```python
from build123d import *

# Parameters (mm, degrees)
F0_W     = 1300
F0_H     = 600
F1_DEPTH = 800
F2_W     = 1220
F2_H     = 80
F3_DEPTH = 800.001
F4_W     = 1220
F4_H     = 200
F5_DEPTH = 800.001
F6_W     = 590
F6_H     = 200
F7_DEPTH = 780


with BuildPart() as f1:
    # F0 (on Front) → F1 (new body)
    with BuildSketch(Plane.XZ):
        Rectangle(F0_W, F0_H)
    extrude(amount=F1_DEPTH)

    # F2 (on face) → F3 (cut, through all)
    with BuildSketch(Plane.XZ.offset(800)):
        with Locations((0, -260)):
            Rectangle(F2_W, F2_H)
    extrude(amount=-F3_DEPTH, mode=Mode.SUBTRACT)

    # F4 (on face) → F5 (cut, through all)
    with BuildSketch(Plane.XZ.offset(800)):
        with Locations((0, 160)):
            Rectangle(F4_W, F4_H)
    extrude(amount=-F5_DEPTH, mode=Mode.SUBTRACT)

    # F6 (on face) → F7 (cut)
    with BuildSketch(Plane.XZ.offset(800)):
        with Locations((-315, -80)):
            Rectangle(F6_W, F6_H)
        with Locations((315, -80)):
            Rectangle(F6_W, F6_H)
    extrude(amount=-F7_DEPTH, mode=Mode.SUBTRACT)


solid = f1.part
```
Source: CAD feature listing. Evaluate the final solid. Frame: model axes, mm. A direction names the side the tool comes from. Coordinates: 2 decimals unless noted, no trailing zeros. Loops run counter-clockwise (first coordinate to the right, second up) from the corner with the lowest first, then second, coordinate; pieces in that order, holes last. Notation, with made-up numbers: M -23,63 L -10,63 A27 cw -10,79 Z; hole C 77.25,-28.75 d5. An arc over 180 degrees is marked long. Use a Markdown table: item, result. Add a question column.
Q1. Section query B-B, the plane z = 231. Return loops of the section in (x, y), and give its area (3 significant figures).
Q2. Draft query along Z for faces 5 (the flat face through (-9, -394, 300)), 6 (the flat face through (630, -394, -300)), 7 (the flat face through (311, -20, -79)), 8 (the flat face through (-610, -406, -261)). Return one class per face: pulls with the +Z half, pulls with the -Z half, needs draft (parallel to the pull), parting line crosses it, or undercut.
Q3. Section query C-C, the plane y = -740.5. Return loops of the section in (x, z), and give its area (3 significant figures).
Q4. Access query for faces 1 (the flat face through (-610, -406, 159)), 2 (the flat face through (20, -415, -81)), 3 (the flat face through (-3, -800, 46)), 4 (the flat face through (-9, -406, -220)). Directions: +Z, -Z, +X, -X, +Y, -Y. A direction counts if a zero-diameter tool reaches every point of the face in a straight line with its end or side. Return the directions, or none.
Q5. Material intervals for L1, parallel to Z at x = 431, y = -731; L2, parallel to X at y = -482, z = -98.5; L3, parallel to X at y = -748, z = 92.5, sorted ascending.
Q6. Section query D-D, the plane z = -69.5. Return loops of the section in (x, y).
Q7. Section query A-A, the plane x = -187. Return loops of the section in (y, z), and give its area (3 significant figures).
Q8. First-contact query: pin 1 (3 mm diameter, centred on x = -182, z = -155.5, fed in from -Y); pin 2 (10 mm diameter, centred on x = 323, y = -558, fed in from -Z). Flat tips, straight axial feed; report the tip coordinate or a pass-through.
Result:
| question | item | result |
|---|---|---|
| 1 | outline | M -650,-800 L -610,-800 L -610,0 L -650,0 Z; M 610,-800 L 650,-800 L 650,0 L 610,0 Z |
| 1 | area | 64,000 mm2 |
| 2 | face 5 | pulls with the +Z half |
| 2 | face 6 | pulls with the -Z half |
| 2 | face 7 | undercut |
| 2 | face 8 | needs draft |
| 3 | outline | M -650,-300 L -610,-300 L -610,-220 L 610,-220 L 610,-300 L 650,-300 L 650,300 L -650,300 Z; hole M -610,-180 L -20,-180 L -20,20 L -610,20 Z; hole M -610,60 L 610,60 L 610,260 L -610,260 Z; hole M 20,-180 L 610,-180 L 610,20 L 20,20 Z |
| 3 | area | 202,000 mm2 |
| 4 | face 1 | +Y, -Y |
| 4 | face 2 | -Y |
| 4 | face 3 | +Z, -Z, +X, -X, -Y |
| 4 | face 4 | -Z, +Y, -Y |
| 5 | L1 | z = -220 to -180, 20 to 60, 260 to 300 |
| 5 | L2 | x = -650 to -610, -20 to 20, 610 to 650 |
| 5 | L3 | x = -650 to -610, 610 to 650 |
| 6 | outline | M -650,-800 L -610,-800 L -610,-20 L -20,-20 L -20,-800 L 20,-800 L 20,-20 L 610,-20 L 610,-800 L 650,-800 L 650,0 L -650,0 Z |
| 7 | outline | M -800,-220 L 0,-220 L 0,60 L -800,60 L -800,20 L -20,20 L -20,-180 L -800,-180 Z; M -800,260 L 0,260 L 0,300 L -800,300 Z |
| 7 | area | 100,000 mm2 |
| 8 | pin 1 | stops at y = -20 |
| 8 | pin 2 | stops at z = -220 |
